Autodesk Inventor part; units mm, degrees
ref_plane "Start Plane" through (0, 0, -150) normal (0, 0, 1) x (1, 0, 0)
ref_plane "End Plane" through (0, 0, 1180) normal (0, 0, 1) x (1, 0, 0)
ref_plane "Work Plane4" through (0, -984.5, 1180) normal (0, 0, 1) x (1, 0, 0)
ref_plane "Start Plane" through (0, 0, -150) normal (0, 0, 1) x (1, 0, 0)
ref_plane "End Plane" through (0, 0, 1180) normal (0, 0, 1) x (1, 0, 0)
sketch "Sketch" plane through (0, 0, 0) normal (0, 0, 1) x (1, 0, 0)
  line L0 (-20, -15.5) -> (-20, 15.5)
  line L1 (-15.5, 20) -> (15.5, 20)
  line L2 (20, 15.5) -> (20, -15.5)
  line L3 (15.5, -20) -> (-15.5, -20)
  arc A0 (-20, -15.5) -> (-15.5, -20) centre (-15.5, -15.5) ccw
  arc A1 (-15.5, 20) -> (-20, 15.5) centre (-15.5, 15.5) ccw
  arc A2 (20, 15.5) -> (15.5, 20) centre (15.5, 15.5) ccw
  arc A3 (15.5, -20) -> (20, -15.5) centre (15.5, -15.5) ccw
  arc A4 (-15.5, 17) -> (-17, 15.5) centre (-15.5, 15.5) ccw
  line L4 (-15.5, 17) -> (15.5, 17)
  arc A5 (17, 15.5) -> (15.5, 17) centre (15.5, 15.5) ccw
  line L5 (17, 15.5) -> (17, -15.5)
  arc A6 (15.5, -17) -> (17, -15.5) centre (15.5, -15.5) ccw
  line L6 (15.5, -17) -> (-15.5, -17)
  arc A7 (-17, -15.5) -> (-15.5, -17) centre (-15.5, -15.5) ccw
  line L7 (-17, -15.5) -> (-17, 15.5)
  line L8 (0, 29.3048) -> (0, -29.3048) construction
  line L9 (-29.3048, 0) -> (29.3048, 0) construction
  dimension "d7" = 4.5
  dimension "d10" = 40
  dimension "d11" = 40
  dimension "d12" = 3
  dimension "d15" = 20
  dimension "d16" = 20
extrude "Body" add sketch "Sketch" along normal up to surface (1330 mm away) from surface at -150
sketch "Sketch3" plane through (0, 0, 0) normal (0, 0, 1) x (1, 0, 0)
  line L0 (0, 0) -> (10, 0)
ref_plane "Work Plane3" through (0, 0, 0) normal (0, -1, 0) x (1, 0, 0)
ref_plane "Work Plane4" through (0, -984.5, 1180) normal (0, 0, 1) x (1, 0, 0)
split "Split1" plane through (0, -984.5, 1180) removes the side toward (0, 0, 1)
sketch "Sketch4" plane through (0, 0, 0) normal (0, -1, 0) x (1, 0, 0)
  line L0 (-2, -150) -> (12, -150)
  line L1 (-2, 1180) -> (12, 1180)
  dimension "d18" = 1330
equation "\"d7\" = G_IR"
equation "\"d10\" = G_H"
equation "\"d11\" = G_W"
equation "\"d12\" = G_T"
equation "\"d15\" = 0.5 * d10"
equation "\"d16\" = 0.5 * d11"
equation "\"d3\" = G_L"
equation "\"G_W\" = 40"
equation "\"G_H\" = 40"
equation "\"G_T\" = 3"
equation "\"G_IR\" = 4.5"
equation "\"G_L\" = d18"
properties part number "ISO 12633-2 - 40x40x3 - 1330" material "Steel, Mild"
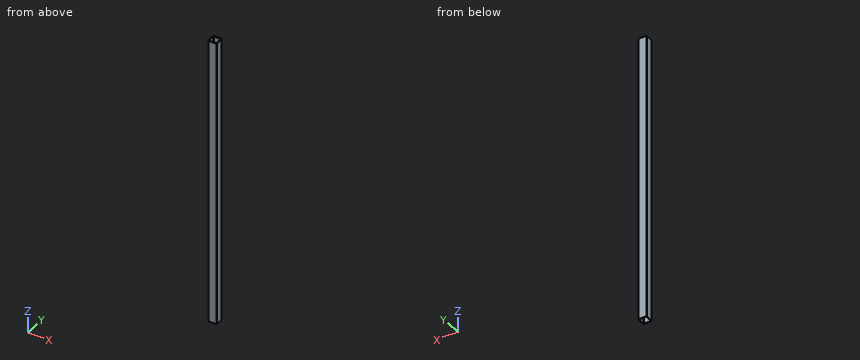
Read the model definition and answer for the solid it produces. Units are mm, in the model's axes. Coordinates: 2 decimals unless noted, no trailing zeros. Loops run counter-clockwise (first coordinate to the right, second up) from the corner with the lowest first, then second, coordinate; pieces in that order, holes last. Notation, with made-up numbers: (74.5, 30.5) -> (80.5, 30.5) arc R24 ccw to (80.5, 57.5) -> close; hole circle Ø2 at (18.5, -32.5). An arc over 180 degrees is marked (long way). Answer in a Markdown table with one row per item.
Item 1: Straight lines are drawn through the part: line 1 along X through (y, z) = (-16, -84); line 2 along X through (y, z) = (14, 870). For each, find the intervals that lie inside material, in ascending order. Write a range as [from, to].
Returned:
| item | result |
|---|---|
| line 1 | x = [-19.97, -16.91], [16.91, 19.97] |
| line 2 | x = [-20, -17], [17, 20] |
Item 2: A cutting plane is placed at C-C on z = 105.5. Determine the outline of the cut face in (x, y).
Returned:
| item | result |
|---|---|
| outline | (-20, -15.5) arc R4.5 ccw to (-15.5, -20) -> (15.5, -20) arc R4.5 ccw to (20, -15.5) -> (20, 15.5) arc R4.5 ccw to (15.5, 20) -> (-15.5, 20) arc R4.5 ccw to (-20, 15.5) -> close; hole (-17, -15.5) arc R1.5 ccw to (-15.5, -17) -> (15.5, -17) arc R1.5 ccw to (17, -15.5) -> (17, 15.5) arc R1.5 ccw to (15.5, 17) -> (-15.5, 17) arc R1.5 ccw to (-17, 15.5) -> close |
Item 3: A cutting plane is placed at A-A on x = -6.5. Determine the outline of the cut face in (y, z), plus the area to 3 significant figures.
Returned:
| item | result |
|---|---|
| outline | (-20, -150) -> (-17, -150) -> (-17, 1180) -> (-20, 1180) -> close; (17, -150) -> (20, -150) -> (20, 1180) -> (17, 1180) -> close |
| area | 7,980 mm^2 |
